from build123d import *

# Parameters (mm, degrees)
RESSALTO_EXTRUS_O1_DEPTH = 6
ESBO_O2_OUTSIDE_W        = 119.66
ESBO_O2_OUTSIDE_H        = 117.678
ESBO_O2_OUTSIDE_R        = 7
CORTE_EXTRUS_O1_DEPTH    = 13
CORTE_EXTRUS_O1_DRAFT    = -75
ESBO_O9_OUTSIDE_W        = 119.66
ESBO_O9_OUTSIDE_H        = 117.678
ESBO_O9_OUTSIDE_R        = 7
CORTE_EXTRUS_O6_DEPTH    = 13
CORTE_EXTRUS_O6_DRAFT    = -75
ESBO_O10_R               = 4
RESSALTO_EXTRUS_O2_DEPTH = 40


with BuildPart() as part:
    # Esboço1 → Ressalto-extrusão1 (new body)
    with BuildSketch(Plane.XY):
        Polygon((3.880998386, 7.090217547), (-4.199809321, 6.906151968), (-8.080807707, -0.184065579), (-3.880998386, -7.090217547), (4.199809321, -6.906151968), (8.080807707, 0.184065579), align=None)
    extrude(amount=RESSALTO_EXTRUS_O1_DEPTH)


with BuildPart() as corte_extrus_o1_tool:
    # Esboço2 outside → Corte-extrusão1 (with draft: the straight prism first)
    with BuildSketch(Plane.XY.offset(6)):
        Rectangle(ESBO_O2_OUTSIDE_W, ESBO_O2_OUTSIDE_H)
        Circle(ESBO_O2_OUTSIDE_R, mode=Mode.SUBTRACT)
    extrude(amount=-CORTE_EXTRUS_O1_DEPTH)
    # Corte-extrusão1: the draft: its side faces are tilted about the plane it starts from
    corte_extrus_o1_sides = [corte_extrus_o1_tool.faces().sort_by_distance(p)[0] for p in [
        (0, -58.839, -0.5),
        (59.83, 0, -0.5),
        (0, 58.839, -0.5),
        (-59.83, 0, -0.5),
        (-7, 0, -0.5),
    ]]
    draft(corte_extrus_o1_sides, Plane.XY.offset(6), CORTE_EXTRUS_O1_DRAFT)


with BuildPart() as part_1:
    add(part.part)

    # Corte-extrusão1: cut by corte_extrus_o1_tool
    add(corte_extrus_o1_tool.part, mode=Mode.SUBTRACT)


with BuildPart() as corte_extrus_o6_tool:
    # Esboço9 outside → Corte-extrusão6 (with draft: the straight prism first)
    with BuildSketch(Plane(origin=(0, 0, 0), x_dir=(-1, 0, 0), z_dir=(0, 0, -1))):
        Rectangle(ESBO_O9_OUTSIDE_W, ESBO_O9_OUTSIDE_H)
        Circle(ESBO_O9_OUTSIDE_R, mode=Mode.SUBTRACT)
    extrude(amount=-CORTE_EXTRUS_O6_DEPTH)
    # Corte-extrusão6: the draft: its side faces are tilted about the plane it starts from
    corte_extrus_o6_sides = [corte_extrus_o6_tool.faces().sort_by_distance(p)[0] for p in [
        (0, -58.839, 6.5),
        (-59.83, 0, 6.5),
        (0, 58.839, 6.5),
        (59.83, 0, 6.5),
        (7, 0, 6.5),
    ]]
    draft(corte_extrus_o6_sides, Plane(origin=(0, 0, 0), x_dir=(-1, 0, 0), z_dir=(0, 0, -1)), CORTE_EXTRUS_O6_DRAFT)


with BuildPart() as part_2:
    add(part_1.part)

    # Corte-extrusão6: cut by corte_extrus_o6_tool
    add(corte_extrus_o6_tool.part, mode=Mode.SUBTRACT)

    # Esboço10 → Ressalto-extrusão2 (add)
    with BuildSketch(Plane(origin=(0, 0, 0), x_dir=(-1, 0, 0), z_dir=(0, 0, -1))):
        with Locations(Location((0, 0, 0), (0, 0, 180))):
            Circle(ESBO_O10_R)
    extrude(amount=RESSALTO_EXTRUS_O2_DEPTH)


solid = part_2.part
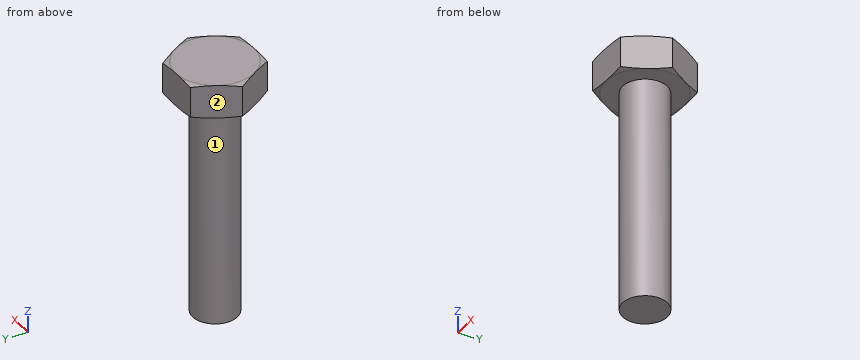
Work out the finished part from the listing and answer in its coordinate system (mm). Face numbers are marked on the shaded views. A direction names the side the tool comes from. Give positions to 0.01 mm unless a question says otherwise; leave off trailing zeros. Loops run counter-clockwise (first coordinate to the right, second up) from the corner with the lowest first, then second, coordinate; pieces in that order, holes last. Notation, with made-up numbers: (88.25, 19) - (101.25, 19) arc R8 ccw to (101.25, 24) - close; hole circle Ø1 at (-39, -36). An arc over 180 degrees is marked (long way). Answer in a Markdown table with one row per item.
(1) Flat-ended cylindrical pins translate along their axes: pin 1 Ø8 at (x, z) = (-1, -10) entering from +Y; pin 2 Ø3 at (x, z) = (-5, -11) entering from +Y; pin 3 Ø3 at (y, z) = (5, -22.5) entering from -X. Find the tip coordinate at first contact, or state that the pin passes through.
Results list:
| item | result |
|---|---|
| pin 1 | stops at y = 4 |
| pin 2 | stops at y = 1.94 |
| pin 3 | stops at x = -1.94 |
(2) Consider L1, parallel to Y at x = 0.25, z = -28.5; L2, parallel to X at y = -1, z = -28; L3, parallel to Z at x = -5.5, y = -2.25. Determine where each line is inside the solid, lowest interval first. Write a range as [from, to].
Results list:
| item | result |
|---|---|
| L1 | y = [-3.99, 3.99] |
| L2 | x = [-3.87, 3.87] |
| L3 | z = [0, 6] |
(3) Section A-A (z = -3) is taken. Give the vertices of the cut face in (x, y).
Results list:
| item | result |
|---|---|
| outline | circle Ø8 at (0, 0) |
(4) A tool of negligible diameter and unlimited length cuts with its end or side. For the marked faces 1 and 2, from which of +Z, -Z, +X, -X, +Y, -Y can it reach the whole face along a straight path? Write none if from no direction.
Results list:
| item | result |
|---|---|
| face 1 | -Z |
| face 2 | +Z, -Z, -X, +Y |
